Source: CAD feature listing. Evaluate the final solid. Frame: model axes, mm. A direction names the side the tool comes from. Give positions to 0.01 mm unless a question says otherwise; leave off trailing zeros. Order: outer loops, then holes, each group sorted by start corner. A loop starts at its lowest first (then second) coordinate and runs counter-clockwise, first axis right, second up. Notation, with made-up numbers: M 59.25,31.25 L 70.25,31.25 A20 ccw 70.25,68.25 Z; hole C -25.5,82 d10. An arc over 180 degrees is marked long. Answer in a Markdown table with one row per item. Add a question column.
(1) Pin query (flat end, axial travel): P1, Ø1.2, axis at x = 67.056, z = 14.605, coming from the +Y side; P2, Ø1.7, axis at y = 7, z = 0.5, coming from the +X side; P3, Ø7, axis at x = -66.5, z = 14.5, coming from the +Y side; P4, Ø1.5, axis at y = 1, z = 3.5, coming from the -X side. Return the tip coordinate at first contact, or that it passes through.
(2) Mould query, pull axis Z, two halves, no side actions, for faces 1 (the face through (-1, 5, 22.225)), 2 (the face through (28.37, 6, 0)), 3 (the face through (0.98, 1.15, -21.14)). Classes: pulls with the +Z half, pulls with the -Z half, needs draft (parallel to the pull), parting line crosses it, or undercut.
(3) Material intervals for line 1 along X through (y, z) = (7.75, -7) (3 decimals); line 2 along Z through (x, y) = (-51.5, 4.25) (3 decimals); line 3 along X through (y, z) = (6.25, 17), sorted ascending.
(4) Section query B-B, the plane x = -58. Return loops of the section in (y, z) (3 decimals), plus the area to 3 significant figures.
(5) Set-up query: faces 4 (the face through (-63.881, 5, -15)), 5 (the face through (-41, 8.636, 0)), 6 (the face through (65.04, 0.66, 15.44)). Return all of +Z, -Z, +X, -X, +Y, -Y with unobstructed straight access to the full face (end or side cutting, diameter ignored); none if empty.
(6) Section query A-A, the plane x = 53. Return loops of the section in (y, z) (3 decimals).
(7) Section query C-C, the plane x = -7.5. Return loops of the section in (y, z) (3 decimals).
from build123d import *

# Parameters (mm, degrees)
SKETCH1_W                                       = 148.082
SKETCH1_H                                       = 44.45
BOSS_EXTRUDE1_DEPTH                             = 6.35
FILLET1_R                                       = 3.81
SHELL1_T                                        = -2.54
SKETCH3_W                                       = 6.35
SKETCH3_H                                       = 7.62
BOSS_EXTRUDE2_DEPTH                             = 4.318
SKETCH5_W                                       = 22.86
SKETCH5_H                                       = 22.86
BOSS_EXTRUDE3_DEPTH                             = 6.096
SKETCH7_W                                       = 19.05
SKETCH7_H                                       = 19.05
CUT_EXTRUDE1_DEPTH                              = 3.302
SKETCH8_W                                       = 21.59
SKETCH8_H                                       = 33.02
BOSS_EXTRUDE4_DEPTH                             = 6.096
SKETCH9_W                                       = 2.54
SKETCH9_H                                       = 35.135780098
BOSS_EXTRUDE5_DEPTH                             = 6.096
SKETCH12_W                                      = 19.05
SKETCH12_H                                      = 30.48
CUT_EXTRUDE2_DEPTH                              = 6.096
CBORE_FOR_1_PAN_HEAD_MACHINE_SCREW3_D           = 2.0574
CBORE_FOR_1_PAN_HEAD_MACHINE_SCREW3_CBORE_D     = 4.36626
CBORE_FOR_1_PAN_HEAD_MACHINE_SCREW3_CBORE_DEPTH = 1.3462


with BuildPart() as part:
    # Sketch1 → Boss-Extrude1 (new body)
    with BuildSketch(Plane(origin=(0, 0, 0), x_dir=(1, 0, 0), z_dir=(0, 1, 0))):
        Rectangle(SKETCH1_W, SKETCH1_H)
    extrude(amount=BOSS_EXTRUDE1_DEPTH)

    # Fillet1
    fillet1_edges = [part.edges().sort_by_distance(p)[0] for p in [
        (0, 0, -22.225),
        (74.041, 0, 0),
        (0, 0, 22.225),
        (-74.041, 0, 0),
        (-74.041, 3.175, -22.225),
        (74.041, 3.175, -22.225),
        (74.041, 3.175, 22.225),
        (-74.041, 3.175, 22.225),
    ]]
    fillet(fillet1_edges, radius=FILLET1_R)

    # Shell1
    shell1_openings = [part.faces().sort_by_distance(p)[0] for p in [
        (0, 6.35, 0),
    ]]
    offset(amount=SHELL1_T, openings=shell1_openings, kind=Kind.INTERSECTION)

    # Sketch3 → Boss-Extrude2 (add)
    with BuildSketch(Plane(origin=(0, 2.54, 0), x_dir=(1, 0, 0), z_dir=(0, 1, 0))):
        with Locations((-67.056, 14.605)):
            Rectangle(SKETCH3_W, SKETCH3_H)
        with Locations((67.056, 14.605)):
            Rectangle(SKETCH3_W, SKETCH3_H)
        with Locations((-67.056, -14.605)):
            Rectangle(SKETCH3_W, SKETCH3_H)
        with Locations((67.056, -14.605)):
            Rectangle(SKETCH3_W, SKETCH3_H)
    extrude(amount=BOSS_EXTRUDE2_DEPTH)

    # Sketch5 → Boss-Extrude3 (add)
    with BuildSketch(Plane(origin=(0, 2.54, 0), x_dir=(1, 0, 0), z_dir=(0, 1, 0))):
        with Locations((-50.8, 0)):
            Rectangle(SKETCH5_W, SKETCH5_H)
    extrude(amount=BOSS_EXTRUDE3_DEPTH)

    # Sketch7 → Cut-Extrude1 (cut)
    with BuildSketch(Plane(origin=(0, 8.636, 0), x_dir=(1, 0, 0), z_dir=(0, 1, 0))):
        with Locations((-50.8, 0)):
            Rectangle(SKETCH7_W, SKETCH7_H)
    extrude(amount=-CUT_EXTRUDE1_DEPTH, mode=Mode.SUBTRACT)

    # Sketch8 → Boss-Extrude4 (add)
    with BuildSketch(Plane(origin=(0, 2.54, 0), x_dir=(1, 0, 0), z_dir=(0, 1, 0))):
        with Locations((49.639483249, 0)):
            Rectangle(SKETCH8_W, SKETCH8_H)
    extrude(amount=BOSS_EXTRUDE4_DEPTH)

    # Sketch9 → Boss-Extrude5 (add)
    with BuildSketch(Plane(origin=(0, 2.54, 0), x_dir=(1, 0, 0), z_dir=(0, 1, 0))):
        with Locations((-34.367719814, 0)):
            Rectangle(SKETCH9_W, SKETCH9_H)
        with Locations((27.100280186, 0)):
            Rectangle(SKETCH9_W, SKETCH9_H)
    extrude(amount=BOSS_EXTRUDE5_DEPTH)

    # Sketch12 → Cut-Extrude2 (cut)
    with BuildSketch(Plane(origin=(0, 8.636, 0), x_dir=(1, 0, 0), z_dir=(0, 1, 0))):
        with Locations((49.639483249, 0)):
            Rectangle(SKETCH12_W, SKETCH12_H)
    extrude(amount=-CUT_EXTRUDE2_DEPTH, mode=Mode.SUBTRACT)

    # CBORE for #1 Pan Head Machine Screw3 (through all)
    with Locations(Plane(origin=(0, 0, 0), x_dir=(-1, 0, 0), z_dir=(0, -1, 0))):
        with Locations((-67.056, 14.605), (-67.056, -14.605), (67.056, -14.605), (67.056, 14.605)):
            CounterBoreHole(CBORE_FOR_1_PAN_HEAD_MACHINE_SCREW3_D / 2, CBORE_FOR_1_PAN_HEAD_MACHINE_SCREW3_CBORE_D / 2, CBORE_FOR_1_PAN_HEAD_MACHINE_SCREW3_CBORE_DEPTH)


solid = part.part
Values follow:
| question | item | result |
|---|---|---|
| 1 | P1 | passes through |
| 1 | P2 | stops at x = 74.04 |
| 1 | P3 | stops at y = 6.86 |
| 1 | P4 | stops at x = -73.44 |
| 2 | face 1 | pulls with the +Z half |
| 2 | face 2 | undercut |
| 2 | face 3 | pulls with the -Z half |
| 3 | line 1 | x = -62.23 to -60.325, -41.275 to -39.37, -35.638 to -33.098, 25.83 to 28.37, 38.844 to 40.114, 59.164 to 60.434 |
| 3 | line 2 | z = -22.225 to -19.685, -11.43 to 11.43, 19.685 to 22.225 |
| 3 | line 3 | x = -74.04 to -71.5, -70.23 to -63.88, -35.64 to -33.1, 25.83 to 28.37, 63.88 to 70.23, 71.5 to 74.04 |
| 4 | outline | M 0,-18.415 A3.81 ccw 3.81,-22.225 L 6.35,-22.225 L 6.35,-19.685 L 3.81,-19.685 A1.27 cw 2.54,-18.415 L 2.54,-11.43 L 8.636,-11.43 L 8.636,-9.525 L 5.334,-9.525 L 5.334,9.525 L 8.636,9.525 L 8.636,11.43 L 2.54,11.43 L 2.54,18.415 A1.27 cw 3.81,19.685 L 6.35,19.685 L 6.35,22.225 L 3.81,22.225 A3.81 ccw 0,18.415 Z |
| 4 | area | 203 mm² |
| 5 | face 4 | +Y |
| 5 | face 5 | +Z, -Z, +X, -X, +Y |
| 5 | face 6 | -Y |
| 6 | outline | M 0,-18.415 A3.81 ccw 3.81,-22.225 L 6.35,-22.225 L 6.35,-19.685 L 3.81,-19.685 A1.27 cw 2.54,-18.415 L 2.54,-16.51 L 8.636,-16.51 L 8.636,-15.24 L 2.54,-15.24 L 2.54,15.24 L 8.636,15.24 L 8.636,16.51 L 2.54,16.51 L 2.54,18.415 A1.27 cw 3.81,19.685 L 6.35,19.685 L 6.35,22.225 L 3.81,22.225 A3.81 ccw 0,18.415 Z |
| 7 | outline | M 0,-18.415 A3.81 ccw 3.81,-22.225 L 6.35,-22.225 L 6.35,-19.685 L 3.81,-19.685 A1.27 cw 2.54,-18.415 L 2.54,18.415 A1.27 cw 3.81,19.685 L 6.35,19.685 L 6.35,22.225 L 3.81,22.225 A3.81 ccw 0,18.415 Z |
